Geometry: final body of the model. Coordinates: model frame, mm. Face numbers are marked on the shaded views. A direction names the side the tool comes from. Round coordinates to 2 decimals unless told otherwise and drop trailing zeros. Loops run counter-clockwise (first coordinate to the right, second up) from the corner with the lowest first, then second, coordinate; pieces in that order, holes last. Notation, with made-up numbers: M 39,-11.75 L 50,-11.75 A28 ccw 50,22.25 Z; hole C 26.5,81 d10. An arc over 180 degrees is marked long. Answer as a JSON object with one key per item and string values.
```python
from build123d import *

# Parameters (mm, degrees)
F0_W      = 38.1
F0_H      = 25.4
F1_DEPTH  = 31.75
F2_W      = 19.05
F2_H      = 12.7
F3_DEPTH  = 25.4
F4_W      = 12.7
F4_H      = 6.35
F5_DEPTH  = 25.4
F6_DEPTH  = 19.05
F7_W      = 12.7
F7_H      = 12.7
F8_DEPTH  = 25.4
F9_W      = 12.7
F9_H      = 12.7
F10_DEPTH = 25.4
F11_W     = 12.7
F11_H     = 12.7
F12_DEPTH = 25.4
F13_W     = 38.1
F13_H     = 12.7
F14_DEPTH = 12.7


with BuildPart() as f1:
    # F0 (on Top) → F1 (new body)
    with BuildSketch(Plane.XY):
        with Locations((-19.05, 2.3111041307)):
            Rectangle(F0_W, F0_H)
    extrude(amount=F1_DEPTH)

    # F2 (on face) → F3 (cut)
    with BuildSketch(Plane.XZ.offset(10.3888958693)):
        Polygon((-38.1, 31.75), (-38.1, 25.4), (-19.05, 25.4), (0, 25.4), (0, 31.75), align=None)
        with Locations((-28.575, 19.05)):
            Rectangle(F2_W, F2_H)
    extrude(amount=-F3_DEPTH, mode=Mode.SUBTRACT)

    # F4 (on face) → F5 (cut)
    with BuildSketch(Plane(origin=(0, 15.0111041307, 0), x_dir=(-1, 0, 0), z_dir=(0, 1, 0))):
        with Locations((19.05, 3.175)):
            Rectangle(F4_W, F4_H)
    extrude(amount=-F5_DEPTH, mode=Mode.SUBTRACT)

    # F6 (add): a face of the model
    f6_faces = [f1.faces().sort_by_distance(p)[0] for p in [
        (-19.05, 2.3111041307, 19.05),
    ]]
    extrude(f6_faces, amount=F6_DEPTH)

    # F7 (on face) → F8 (cut)
    with BuildSketch(Plane(origin=(0, 0, 0), x_dir=(1, 0, 0), z_dir=(0, 0, -1))):
        with Locations((-31.75, -8.6611041307)):
            Rectangle(F7_W, F7_H)
    extrude(amount=-F8_DEPTH, mode=Mode.SUBTRACT)

    # F9 (on face) → F10 (cut)
    with BuildSketch(Plane(origin=(0, 0, 0), x_dir=(1, 0, 0), z_dir=(0, 0, -1))):
        with Locations((-6.35, -8.6611041307)):
            Rectangle(F9_W, F9_H)
    extrude(amount=-F10_DEPTH, mode=Mode.SUBTRACT)

    # F11 (on face) → F12 (cut)
    with BuildSketch(Plane(origin=(0, 0, 6.35), x_dir=(1, 0, 0), z_dir=(0, 0, -1))):
        with Locations((-19.05, -8.6611041307)):
            Rectangle(F11_W, F11_H)
    extrude(amount=-F12_DEPTH, mode=Mode.SUBTRACT)

    # F13 (on face) → F14 (join)
    with BuildSketch(Plane(origin=(0, 2.3111041307, 0), x_dir=(-1, 0, 0), z_dir=(0, 1, 0))):
        with Locations((19.05, 19.05)):
            Rectangle(F13_W, F13_H)
    extrude(amount=F14_DEPTH)


solid = f1.part
```
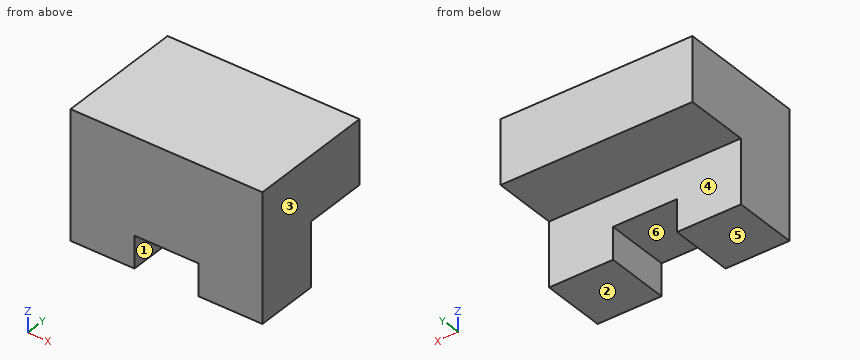
1) Cut plane B-B on x = -5. Return the cut outline in (y, z).
Geometry results:
{"outline": "M -10.39,0 L 2.31,0 L 2.31,12.7 L 15.01,12.7 L 15.01,25.4 L -10.39,25.4 Z"}
2) Cut plane D-D on x = -24. Return the cut outline in (y, z).
Geometry results:
{"outline": "M -10.39,6.35 L 2.31,6.35 L 2.31,12.7 L 15.01,12.7 L 15.01,25.4 L -10.39,25.4 Z"}
3) Line query: probe 1 along Z at (x, y) = (-32.5, 7.75); probe 2 along Y at (x, z) = (-9, 8.5). Output: solid intervals per line, ascending.
Geometry results:
{"probe 1": "12.7 to 25.4", "probe 2": "-10.39 to 2.31"}
4) Cut plane A-A on z = 4. Return the cut outline in (x, y), and give its area (3 significant figures).
Geometry results:
{"outline": "M -38.1,-10.39 L -25.4,-10.39 L -25.4,2.31 L -38.1,2.31 Z; M -12.7,-10.39 L 0,-10.39 L 0,2.31 L -12.7,2.31 Z", "area": "323 mm2"}
5) First-contact query: pin 1 (3 mm diameter, centred on x = -18, y = 0, fed in from -Z); pin 2 (4 mm diameter, centred on x = -25.5, z = 5, fed in from +Y). Flat tips, straight axial feed; report the tip coordinate or a pass-through.
Geometry results:
{"pin 1": "z = 6.35", "pin 2": "y = 2.31"}
6) Cut plane C-C on y = -6.5. Return the cut outline in (x, z).
Geometry results:
{"outline": "M -38.1,0 L -25.4,0 L -25.4,6.35 L -12.7,6.35 L -12.7,0 L 0,0 L 0,25.4 L -38.1,25.4 Z"}
7) Pull-direction query (X, two-part tool) for the marked faces 1, 2 and 3; classes: +X half, -X half, draft (parallel to the pull), parting line (faces both ways), or undercut.
Geometry results:
{"face 1": "undercut", "face 2": "draft", "face 3": "+X half"}
8) Set-up query: the marked faces 4, 5 and 6. Return all of +Z, -Z, +X, -X, +Y, -Y with unobstructed straight access to the full face (end or side cutting, diameter ignored); none if empty.
Geometry results:
{"face 4": "-Z, +X, -X, +Y", "face 5": "-Z, +X, -X, +Y, -Y", "face 6": "-Z, +Y, -Y"}
